```python
from build123d import *

# Parameters (mm, degrees)
EXTRUDE_1_DEPTH     = 4
EXTRUDE_2_DEPTH     = 4
SKETCH_3_R          = 1.25
CUT_EXTRUDE_1_DEPTH = 15
CUT_EXTRUDE_2_DEPTH = 0.2


with BuildPart() as part:
    # 草图1 → 凸台-拉伸1 (new body)
    with BuildSketch(Plane(origin=(0, 0, 0), x_dir=(1, 0, 0), z_dir=(0, 1, 0))):
        with BuildLine():
            Line((-27.00005461, -31.987363475), (27.00005461, -31.987363475))
            ThreePointArc((27.00005461, -31.987363475), (29.112398272, -31.112402082), (29.987359665, -29.00005842))
            Line((29.987359665, -29.00005842), (29.987359665, 29.00005842))
            ThreePointArc((29.987359665, 29.00005842), (29.112398272, 31.112402082), (27.00005461, 31.987363475))
            Line((27.00005461, 31.987363475), (-27.00005461, 31.987363475))
            ThreePointArc((-27.00005461, 31.987363475), (-29.112398272, 31.112402082), (-29.987359665, 29.00005842))
            Line((-29.987359665, 29.00005842), (-29.987359665, -29.00005842))
            ThreePointArc((-29.987359665, -29.00005842), (-29.112398272, -31.112402082), (-27.00005461, -31.987363475))
        make_face()
    extrude(amount=EXTRUDE_1_DEPTH)

    # 草图2 → 凸台-拉伸2 (add)
    with BuildSketch(Plane.XZ):
        with BuildLine():
            Line((-21.987359665, 23.987363475), (-21.987359665, 31.987363475))
            Line((-21.987359665, 31.987363475), (-27.00005461, 31.987363475))
            ThreePointArc((-27.00005461, 31.987363475), (-29.112398272, 31.112402082), (-29.987359665, 29.00005842))
            Line((-29.987359665, 29.00005842), (-29.987359665, 23.987363475))
            Line((-29.987359665, 23.987363475), (-21.987359665, 23.987363475))
        make_face()
        with BuildLine():
            Line((21.987359665, -23.987363475), (21.987359665, -31.987363475))
            Line((21.987359665, -31.987363475), (27.00005461, -31.987363475))
            ThreePointArc((27.00005461, -31.987363475), (29.112398272, -31.112402082), (29.987359665, -29.00005842))
            Line((29.987359665, -29.00005842), (29.987359665, -23.987363475))
            Line((29.987359665, -23.987363475), (21.987359665, -23.987363475))
        make_face()
        with BuildLine():
            Line((21.987359665, 23.987363475), (29.987359665, 23.987363475))
            Line((29.987359665, 23.987363475), (29.987359665, 29.00005842))
            ThreePointArc((29.987359665, 29.00005842), (29.112398272, 31.112402082), (27.00005461, 31.987363475))
            Line((27.00005461, 31.987363475), (21.987359665, 31.987363475))
            Line((21.987359665, 31.987363475), (21.987359665, 23.987363475))
        make_face()
        with BuildLine():
            Line((-29.987359665, -23.987363475), (-29.987359665, -29.00005842))
            ThreePointArc((-29.987359665, -29.00005842), (-29.112398272, -31.112402082), (-27.00005461, -31.987363475))
            Line((-27.00005461, -31.987363475), (-21.987359665, -31.987363475))
            Line((-21.987359665, -31.987363475), (-21.987359665, -23.987363475))
            Line((-21.987359665, -23.987363475), (-29.987359665, -23.987363475))
        make_face()
    extrude(amount=EXTRUDE_2_DEPTH)

    # 草图3 → 切除-拉伸1 (cut)
    with BuildSketch(Plane.XZ.offset(4)):
        with Locations((-27.00005461, 29.00005842)):
            Circle(SKETCH_3_R)
        with Locations((27.00005461, 29.00005842)):
            Circle(SKETCH_3_R)
        with Locations((27.00005461, -29.00005842)):
            Circle(SKETCH_3_R)
        with Locations((-27.00005461, -29.00005842)):
            Circle(SKETCH_3_R)
    extrude(amount=-CUT_EXTRUDE_1_DEPTH, mode=Mode.SUBTRACT)

    # 草图5 → 切除-拉伸2 (cut)
    with BuildSketch(Plane(origin=(0, 4, 0), x_dir=(1, 0, 0), z_dir=(0, 1, 0))):
        with BuildLine():
            ThreePointArc((-24.510212589, -22.489370571), (-23.924426151, -23.903584133), (-22.510212589, -24.489370571))
            Line((-22.510212589, -24.489370571), (23.489787411, -24.489370571))
            Line((23.489787411, -24.489370571), (23.489787411, 23.510629429))
            ThreePointArc((23.489787411, 23.510629429), (22.904000974, 24.924842991), (21.489787411, 25.510629429))
            Line((21.489787411, 25.510629429), (-22.510212589, 25.510629429))
            ThreePointArc((-22.510212589, 25.510629429), (-23.924426151, 24.924842991), (-24.510212589, 23.510629429))
            Line((-24.510212589, 23.510629429), (-24.510212589, -22.489370571))
        make_face()
        with BuildLine():
            Line((-21.404655137, -0.688500192), (-15.457204068, -0.688500192))
            ThreePointArc((-15.457204068, -0.688500192), (-15.242140256, -0.766165613), (-15.126321966, -0.963321604))
            Line((-15.126321966, -0.963321604), (-12.93890785, -12.678969469))
            ThreePointArc((-12.93890785, -12.678969469), (-13.010855373, -12.95581187), (-13.269789952, -13.077348057))
            ThreePointArc((-13.269789952, -13.077348057), (-13.425801703, -13.039009509), (-13.546274154, -12.932727342))
            Line((-13.546274154, -12.932727342), (-21.681139339, -1.217079478))
            ThreePointArc((-21.681139339, -1.217079478), (-21.702916589, -0.869088442), (-21.404655137, -0.688500192))
        make_face(mode=Mode.SUBTRACT)
        with BuildLine():
            Line((-9.512596077, -16.472848359), (-2.571281975, -4.734690874))
            ThreePointArc((-2.571281975, -4.734690874), (-2.248646777, -4.571034999), (-1.964018884, -4.794336767))
            Line((-1.964018884, -4.794336767), (3.140150939, -19.305798562))
            ThreePointArc((3.140150939, -19.305798562), (3.097295639, -19.61204324), (2.822620241, -19.754084802))
            ThreePointArc((2.822620241, -19.754084802), (2.784616416, -19.75193251), (2.7470986, -19.745503158))
            Line((2.7470986, -19.745503158), (-9.298385325, -16.972198847))
            ThreePointArc((-9.298385325, -16.972198847), (-9.53220226, -16.77688017), (-9.512596077, -16.472848359))
        make_face(mode=Mode.SUBTRACT)
        with BuildLine():
            Line((-12.041068111, -0.688500192), (-5.131124443, -0.688500192))
            ThreePointArc((-5.131124443, -0.688500192), (-4.847891187, -0.843225283), (-4.825045876, -1.165155435))
            Line((-4.825045876, -1.165155435), (-10.329425017, -13.194497943))
            ThreePointArc((-10.329425017, -13.194497943), (-10.453628675, -13.337675957), (-10.635503584, -13.391042701))
            ThreePointArc((-10.635503584, -13.391042701), (-10.859278656, -13.305887083), (-10.969829102, -13.093506855))
            Line((-10.969829102, -13.093506855), (-12.375393629, -1.064164346))
            ThreePointArc((-12.375393629, -1.064164346), (-12.292512493, -0.80132512), (-12.041068111, -0.688500192))
        make_face(mode=Mode.SUBTRACT)
        with BuildLine():
            Line((9.36207412, -1.111559506), (5.109122277, -17.113456876))
            ThreePointArc((5.109122277, -17.113456876), (4.988995356, -17.293832498), (4.783815734, -17.363597563))
            ThreePointArc((4.783815734, -17.363597563), (4.581434131, -17.295960844), (4.460386024, -17.120232659))
            Line((4.460386024, -17.120232659), (-0.152481619, -1.118335289))
            ThreePointArc((-0.152481619, -1.118335289), (-0.098015191, -0.822718589), (0.17094809, -0.688500192))
            Line((0.17094809, -0.688500192), (9.036767577, -0.688500192))
            ThreePointArc((9.036767577, -0.688500192), (9.303602512, -0.81992057), (9.36207412, -1.111559506))
        make_face(mode=Mode.SUBTRACT)
        with BuildLine():
            Line((12.808517611, -0.688500192), (21.484169915, -0.688500192))
            ThreePointArc((21.484169915, -0.688500192), (21.775984057, -0.857338258), (21.775051109, -1.194474604))
            Line((21.775051109, -1.194474604), (15.823663685, -11.415302329))
            ThreePointArc((15.823663685, -11.415302329), (15.793013116, -11.45942167), (15.755733936, -11.498102884))
            Line((15.755733936, -11.498102884), (7.668279808, -18.648335147))
            ThreePointArc((7.668279808, -18.648335147), (7.564528755, -18.710947136), (7.445328364, -18.732760181))
            ThreePointArc((7.445328364, -18.732760181), (7.174474873, -18.596004987), (7.123708261, -18.296862298))
            Line((7.123708261, -18.296862298), (12.486897508, -0.92580231))
            ThreePointArc((12.486897508, -0.92580231), (12.608672805, -0.754246701), (12.808517611, -0.688500192))
        make_face(mode=Mode.SUBTRACT)
        with BuildLine():
            Line((-21.681139339, 1.332693738), (-13.546274154, 13.048341603))
            ThreePointArc((-13.546274154, 13.048341603), (-13.14002845, 13.166944855), (-12.93890785, 12.794583729))
            Line((-12.93890785, 12.794583729), (-15.126321966, 1.078935865))
            ThreePointArc((-15.126321966, 1.078935865), (-15.242140256, 0.881779873), (-15.457204068, 0.804114453))
            Line((-15.457204068, 0.804114453), (-21.404655137, 0.804114453))
            ThreePointArc((-21.404655137, 0.804114453), (-21.702916589, 0.984702702), (-21.681139339, 1.332693738))
        make_face(mode=Mode.SUBTRACT)
        with BuildLine():
            Line((-12.375393629, 1.179778607), (-10.969829102, 13.209121115))
            ThreePointArc((-10.969829102, 13.209121115), (-10.68793709, 13.502547995), (-10.329425017, 13.310112203))
            Line((-10.329425017, 13.310112203), (-4.825045876, 1.280769695))
            ThreePointArc((-4.825045876, 1.280769695), (-4.847891187, 0.958839543), (-5.131124443, 0.804114453))
            Line((-5.131124443, 0.804114453), (-12.041068111, 0.804114453))
            ThreePointArc((-12.041068111, 0.804114453), (-12.292512493, 0.916939381), (-12.375393629, 1.179778607))
        make_face(mode=Mode.SUBTRACT)
        with BuildLine():
            Line((-2.571281975, 4.850305134), (-9.512596077, 16.588462619))
            ThreePointArc((-9.512596077, 16.588462619), (-9.53220226, 16.89249443), (-9.298385325, 17.087813107))
            Line((-9.298385325, 17.087813107), (2.7470986, 19.861117418))
            ThreePointArc((2.7470986, 19.861117418), (3.073572684, 19.75742568), (3.140150939, 19.421412823))
            Line((3.140150939, 19.421412823), (-1.964018884, 4.909951027))
            ThreePointArc((-1.964018884, 4.909951027), (-2.086991143, 4.746961869), (-2.281549581, 4.685037267))
            ThreePointArc((-2.281549581, 4.685037267), (-2.448326624, 4.729259125), (-2.571281975, 4.850305134))
        make_face(mode=Mode.SUBTRACT)
        with BuildLine():
            Line((9.036767577, 0.804114453), (0.17094809, 0.804114453))
            ThreePointArc((0.17094809, 0.804114453), (-0.098015191, 0.93833285), (-0.152481619, 1.233949549))
            Line((-0.152481619, 1.233949549), (4.460386024, 17.235846919))
            ThreePointArc((4.460386024, 17.235846919), (4.78733119, 17.479193465), (5.109122277, 17.229071137))
            Line((5.109122277, 17.229071137), (9.36207412, 1.227173766))
            ThreePointArc((9.36207412, 1.227173766), (9.303602512, 0.93553483), (9.036767577, 0.804114453))
        make_face(mode=Mode.SUBTRACT)
        with BuildLine():
            Line((21.484169915, 0.804114453), (12.808517611, 0.804114453))
            ThreePointArc((12.808517611, 0.804114453), (12.608672805, 0.869860962), (12.486897508, 1.04141657))
            Line((12.486897508, 1.04141657), (7.123708261, 18.412476559))
            ThreePointArc((7.123708261, 18.412476559), (7.262798457, 18.794586027), (7.668279808, 18.763949407))
            Line((7.668279808, 18.763949407), (15.755733936, 11.613717144))
            ThreePointArc((15.755733936, 11.613717144), (15.793013116, 11.57503593), (15.823663685, 11.53091659))
            Line((15.823663685, 11.53091659), (21.775051109, 1.310088864))
            ThreePointArc((21.775051109, 1.310088864), (21.775984057, 0.972952518), (21.484169915, 0.804114453))
        make_face(mode=Mode.SUBTRACT)
    extrude(amount=-CUT_EXTRUDE_2_DEPTH, mode=Mode.SUBTRACT)


solid = part.part
```
Verification items for the finished model (mm, model axes). A direction names the side the tool comes from. Coordinates: 2 decimals unless noted, no trailing zeros. Write each loop counter-clockwise with the first axis right and the second up, starting at its lowest first coordinate (ties: lowest second). Pieces come first, ordered by that corner, then holes. Notation, with made-up numbers: M 28,20 L 59,20 A21 cw 59,40 Z; hole C -38,-38 d6. An arc over 180 degrees is marked long. Answer as a JSON object with one key per item and string values. Group by question number.
(1) Material ranges on line 1 (Z direction, x = -27, y = 1); line 2 (Z direction, x = -26, y = 0.75); line 3 (Y direction, x = -27, z = -19), recorded low to high.
(2) Release check for a two-part mould opening along Z. For faces 1 (the face through (-9, 4, 6)), 2 (the face through (27.577, -0.056, -30.109)) record: +Z half, -Z half, draft (parallel to the pull), parting line (faces both ways), or undercut.
(3) Tool access check on faces 3 (the face through (21.987, -2, -28)), 4 (the face through (26, -4, -28)). Record the directions out of +Z, -Z, +X, -X, +Y, -Y that give a thin tool (end or side, any length) a straight path to the whole face; none if there is none.
(4) Cross-section at C-C, the plane z = 20.5. Record the cut outline in (x, y).
(5) Gauge pin test, flat ends, axial feed: pin 1 (1 mm diameter, centred on x = 8.5, z = 6.5, fed in from -Y); pin 2 (1.5 mm diameter, centred on x = 27, z = -29, fed in from -Y). Record the tip position at first contact, or that the pin passes through.
(6) Cross-section at B-B, the plane x = 24.5. Record the cut outline in (y, z).
(7) Cross-section at D-D, the plane z = -2.5. Record the cut outline in (x, y).
(8) Cross-section at A-A, the plane y = -2.75. Record the cut outline in (x, z), and give its area (3 significant figures).
Reply:
{
 "1": {"line 1": "-31.99 to -30.25, -27.75 to 27.75, 30.25 to 31.99", "line 2": "-31.99 to -29.75, -28.25 to 28.25, 29.75 to 31.99", "line 3": "0 to 4"},
 "2": {"face 1": "draft", "face 2": "undercut"},
 "3": {"face 3": "+Z, -Z, -Y", "face 4": "+Z, -Z, +X, -X, -Y"},
 "4": {"outline": "M -29.99,0 L 29.99,0 L 29.99,4 L 23.49,4 L 23.49,3.8 L -24.51,3.8 L -24.51,4 L -29.99,4 Z"},
 "5": {"pin 1": "y = 0", "pin 2": "through"},
 "6": {"outline": "M -4,-31.99 L 4,-31.99 L 4,31.99 L -4,31.99 L -4,23.99 L 0,23.99 L 0,-23.99 L -4,-23.99 Z"},
 "7": {"outline": "M -29.99,0 L 29.99,0 L 29.99,4 L 23.49,4 L 23.49,3.8 L 21.08,3.8 L 21.08,4 L 12.04,4 L 12.04,3.8 L 9.02,3.8 L 9.02,4 L 0.21,4 L 0.21,3.8 L -5.38,3.8 L -5.38,4 L -12.22,4 L -12.22,3.8 L -14.86,3.8 L -14.86,4 L -20.87,4 L -20.87,3.8 L -24.51,3.8 L -24.51,4 L -29.99,4 Z"},
 "8": {"outline": "M -29.99,-29 A2.99 ccw -27,-31.99 L -21.99,-31.99 L -21.99,-23.99 L -29.99,-23.99 Z; M -29.99,23.99 L -21.99,23.99 L -21.99,31.99 L -27,31.99 A2.99 ccw -29.99,29 Z; M 21.99,-31.99 L 27,-31.99 A2.99 ccw 29.99,-29 L 29.99,-23.99 L 21.99,-23.99 Z; M 21.99,23.99 L 29.99,23.99 L 29.99,29 A2.99 ccw 27,31.99 L 21.99,31.99 Z; hole C -27,-29 d2.5; hole C -27,29 d2.5; hole C 27,-29 d2.5; hole C 27,29 d2.5", "area": "229 mm²"}
}
